For this review, take the finished solid that the model builds, in its own axes (mm). A direction names the side the tool comes from. Coordinates: 2 decimals unless noted, no trailing zeros. Loops run counter-clockwise (first coordinate to the right, second up) from the corner with the lowest first, then second, coordinate; pieces in that order, holes last. Notation, with made-up numbers: (-27, -10) - (-5, -10) arc R10 ccw to (-5, 6) - close; hole circle Ø10 at (-20, 89). An arc over 180 degrees is marked (long way). Answer as a JSON object with one key per item and string values. Group by question number.
Item 1: To check wall thickness, follow line 1 (Y direction, x = 4, z = 10.25); line 2 (Y direction, x = 44.5, z = 8.25); line 3 (Y direction, x = -3.5, z = 8). State the ranges of each line that lie inside material, in increasing order.
Item 2: Tool access review of faces 5 (the flat face through (18.096, 40, 3)), 6 (the flat face through (13, 26.5, 5)), 7 (the cylindrical face through (-2.45, 5.83, 5.42)): name each direction out of +Z, -Z, +X, -X, +Y, -Y from which nothing blocks a thin tool from reaching the whole face with its end or side.
Item 3: Mouldability with a two-part tool opening along X and no side actions: class faces 1 (the flat face through (40.4, 26.4, 0)), 2 (the flat face through (20, 0, 5)), 3 (the flat face through (32.62, 36.99, -0.31)), 4 (the cylindrical face through (51.91, 4.7, 4.59)) as released by +X, released by -X, zero draft, split by the parting line, or undercut.
Item 4: Clearance check with flat-ended pins moving along their axes: pin 1 (1.3 mm diameter, centred on x = 44.5, y = 15.5, fed in from +Z); pin 2 (6 mm diameter, centred on y = 38, z = 0.5, fed in from +X); pin 3 (5 mm diameter, centred on x = 25.5, z = 6, fed in from +Y). State where each tip first meets the part, or that it passes through.
Item 5: We need section B-B (z = 8.75). Give the boundary of the cut face in (x, y).
Item 6: We need section A-A (y = 10.5). Give the boundary of the cut face in (x, z).
from build123d import *

# Parameters (mm, degrees)
SKETCH1_R               = 1.1
SKETCH1_W               = 41
SKETCH1_H               = 21
BOSS_EXTRUDE1_DEPTH     = 11
SKETCH2_R               = 9.000000034
BOSS_EXTRUDE2_DEPTH     = 2
BOSS_EXTRUDE3_DEPTH     = 10
BOSS_EXTRUDE4_DEPTH     = 26
SKETCH6_R               = 15.25
CUT_EXTRUDE1_DEPTH      = 11.0000001
SKETCH8_R               = 2
CUT_EXTRUDE3_DEPTH      = 33.905944515
CUT_EXTRUDE3_DEPTH_BACK = 30.994912665
SKETCH11_R              = 3.875
SKETCH11_R_2            = 2
CUT_EXTRUDE4_DEPTH      = 15.37
BOSS_EXTRUDE6_DEPTH     = 1


with BuildPart() as part:
    # Sketch1 → Boss-Extrude1 (new body)
    with BuildSketch(Plane.XY):
        with BuildLine():
            Line((4, -5.500000004), (37, -5.500000004))
            ThreePointArc((37, -5.500000004), (53.000000004, 10.5), (37, 26.500000004))
            Line((37, 26.500000004), (4, 26.500000004))
            ThreePointArc((4, 26.500000004), (-12.000000004, 10.5), (4, -5.500000004))
        make_face()
        with Locations((-3.5, 15.5)):
            Circle(SKETCH1_R, mode=Mode.SUBTRACT)
        with Locations((-3.5, 5.5)):
            Circle(SKETCH1_R, mode=Mode.SUBTRACT)
        with Locations((44.5, 5.5)):
            Circle(SKETCH1_R, mode=Mode.SUBTRACT)
        with Locations((44.5, 15.5)):
            Circle(SKETCH1_R, mode=Mode.SUBTRACT)
        with Locations((20.5, 10.5)):
            Rectangle(SKETCH1_W, SKETCH1_H, mode=Mode.SUBTRACT)
    extrude(amount=BOSS_EXTRUDE1_DEPTH)

    # Sketch2 → Boss-Extrude2 (add)
    with BuildSketch(Plane.XY):
        with BuildLine():
            Line((37, 26.500000004), (4, 26.500000004))
            ThreePointArc((4, 26.500000004), (-12.000000004, 10.5), (4, -5.500000004))
            Line((4, -5.500000004), (37, -5.500000004))
            ThreePointArc((37, -5.500000004), (53.000000004, 10.5), (37, 26.500000004))
        make_face()
        with Locations((30.749999966, 10.5)):
            Circle(SKETCH2_R, mode=Mode.SUBTRACT)
    extrude(amount=-BOSS_EXTRUDE2_DEPTH)

    # Sketch3 → Boss-Extrude3 (add)
    with BuildSketch(Plane.XY):
        with BuildLine():
            Line((37, 26.500000004), (18.095900106, 26.500000004))
            Line((18.095900106, 26.500000004), (18.095900106, 46.500000004))
            Line((18.095900106, 46.500000004), (44.095900176, 46.500000004))
            Line((44.095900176, 46.500000004), (44.095900176, 27.744899316))
            ThreePointArc((44.095900176, 27.744899316), (46.289330037, 24.381962762), (48.82982939, 21.272888969))
            ThreePointArc((48.82982939, 21.272888969), (43.466597892, 25.134996134), (37, 26.500000004))
        make_face()
    extrude(amount=BOSS_EXTRUDE3_DEPTH)

    # Sketch5 → Boss-Extrude4 (add)
    with BuildSketch(Plane(origin=(44.095900176, 0, 0), x_dir=(0, 0, -1), z_dir=(1, 0, 0))):
        with BuildLine():
            Line((0, 26.737992109), (-10, 46.500000004))
            ThreePointArc((-10, 46.500000004), (0.647802696, 48.386011996), (10, 53.814561439))
            add(Edge.make_bspline(
                [(0, 26.737992109), (5.263715072, 40.18126942), (10, 53.814561439)],
                knots=[0, 0, 0, 1, 1, 1], degree=2))
        make_face()
    extrude(amount=-BOSS_EXTRUDE4_DEPTH)

    # Sketch6 → Cut-Extrude1 (cut, through all)
    with BuildSketch(Plane.XY):
        with Locations((34.595900106, 64.15000003)):
            Circle(SKETCH6_R)
    extrude(amount=-CUT_EXTRUDE1_DEPTH, mode=Mode.SUBTRACT)

    # Sketch8 → Cut-Extrude3 (cut, two sides)
    with BuildSketch(Plane(origin=(0, 23.381689927, 7.597171588), x_dir=(-1, 0, 0), z_dir=(0, -0.951056516, -0.309016994))) as cut_extrude3_sk:
        with Locations((-32.562075151, 13.880413242)):
            Circle(SKETCH8_R)
    extrude(amount=CUT_EXTRUDE3_DEPTH, mode=Mode.SUBTRACT)
    extrude(cut_extrude3_sk.sketch, amount=-CUT_EXTRUDE3_DEPTH_BACK, mode=Mode.SUBTRACT)

    # Sketch11 → Cut-Extrude4 (cut)
    with BuildSketch(Plane(origin=(0, 33.367783426, 10.841850055), x_dir=(-1, 0, 0), z_dir=(0, -0.951056516, -0.309016994))):
        with Locations((-32.562075151, 13.880413242)):
            Circle(SKETCH11_R)
        with Locations((-32.562075151, 13.880413242)):
            Circle(SKETCH11_R_2, mode=Mode.SUBTRACT)
    extrude(amount=CUT_EXTRUDE4_DEPTH, mode=Mode.SUBTRACT)

    # Sketch12 → Boss-Extrude6 (add)
    with BuildSketch(Plane.XY.offset(10)):
        with BuildLine():
            Line((44.095900176, 27.744899316), (44.095900176, 46.500000004))
            Line((44.095900176, 46.500000004), (18.095900106, 46.500000004))
            Line((18.095900106, 46.500000004), (18.095900106, 26.500000004))
            Line((18.095900106, 26.500000004), (37, 26.500000004))
            ThreePointArc((37, 26.500000004), (43.466597892, 25.134996134), (48.82982939, 21.272888969))
            ThreePointArc((48.82982939, 21.272888969), (46.289330037, 24.381962762), (44.095900176, 27.744899316))
        make_face()
    extrude(amount=BOSS_EXTRUDE6_DEPTH)


solid = part.part
Check sheet entries:
{
 "1": {"line 1": "y = -5.5 to 0, 21 to 26.5", "line 2": "y = -3.63 to 4.4, 6.6 to 14.4, 16.6 to 27.06", "line 3": "y = -3.63 to 4.4, 6.6 to 14.4, 16.6 to 24.63"},
 "2": {"face 5": "+Z, -Z, -X, +Y", "face 6": "-Z, -X", "face 7": "+Z"},
 "3": {"face 1": "zero draft", "face 2": "undercut", "face 3": "undercut", "face 4": "released by +X"},
 "4": {"pin 1": "stops at z = 0", "pin 2": "stops at x = 44.1", "pin 3": "stops at y = 47.19"},
 "5": {"outline": "(4, -5.5) - (37, -5.5) arc R16 ccw to (48.83, 21.27) arc R37.49 cw to (44.1, 27.74) - (44.1, 46.53) - (18.1, 46.53) - (18.1, 26.5) - (4, 26.5) arc R16 ccw to start; hole circle Ø2.2 at (-3.5, 5.5); hole circle Ø2.2 at (-3.5, 15.5); hole (0, 0) - (41, 0) - (41, 21) - (0, 21) - close; hole circle Ø2.2 at (44.5, 5.5); hole circle Ø2.2 at (44.5, 15.5)"},
 "6": {"outline": "(-12, -2) - (21.75, -2) - (21.75, 0) - (0, 0) - (0, 11) - (-12, 11) - close; (39.75, -2) - (53, -2) - (53, 11) - (41, 11) - (41, 0) - (39.75, 0) - close"}
}
